For this review, take the finished solid that the model builds, in its own axes (mm). Face numbers are marked on the shaded views. Round coordinates to 2 decimals unless told otherwise and drop trailing zeros. Loops run counter-clockwise (first coordinate to the right, second up) from the corner with the lowest first, then second, coordinate; pieces in that order, holes last.
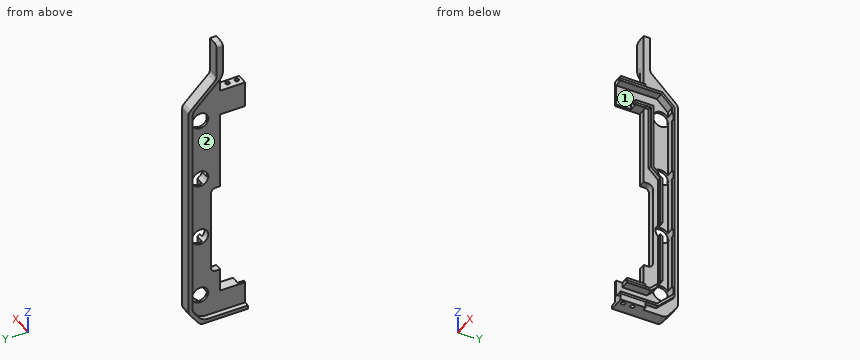
```python
from build123d import *

# Parameters (mm, degrees)
BOSS_EXTRUDE1_DEPTH          = 25
CUT_EXTRUDE1_DEPTH           = 4
FILLET1_R                    = 4
FILLET2_R                    = 10
FILLET3_R                    = 5
FILLET4_R                    = 3
BOSS_EXTRUDE2_DEPTH          = 3
BOSS_EXTRUDE2_DEPTH_BACK     = 3
FILLET5_R                    = 3
SKETCH6_W                    = 13
SKETCH6_H                    = 14
BOSS_EXTRUDE3_DEPTH          = 20
BOSS_EXTRUDE4_DEPTH          = 20
SKETCH9_W                    = 13
SKETCH9_H                    = 2
BOSS_EXTRUDE5_DEPTH          = 8
SKETCH7_W                    = 13
SKETCH7_H                    = 2
CUT_EXTRUDE2_DEPTH           = 5
SKETCH11_R                   = 1.6
CUT_EXTRUDE3_DEPTH           = 19
CUT_EXTRUDE4_START           = -2
SKETCH12_R                   = 1.6
CUT_EXTRUDE4_DEPTH           = 2
CUT_EXTRUDE5_DEPTH           = 6.5
CUT_EXTRUDE5_DEPTH_BACK      = 6.5
CUT_EXTRUDE7_DEPTH           = 247.814201374
BOSS_EXTRUDE6_DEPTH          = 6.5
BOSS_EXTRUDE8_DEPTH          = 3.5
MAKE_THIS_A_SQUARE_OR_SMTH_R = 6.5
CUT_EXTRUDE8_DEPTH           = 134.148413434


with BuildPart() as part:
    # Sketch1 → Boss-Extrude1 (new body)
    with BuildSketch(Plane(origin=(0, 0, 0), x_dir=(0, 0, -1), z_dir=(1, 0, 0))):
        Polygon((0, 0), (-130, 0), (-130, 5), (-100.000366453, 5.148280317), (-77.868517379, 27.5), (101.088229162, 27.5), (114, 18), (114, 0), (74, 0), (74, 7.5), (0, 7.5), align=None)
    extrude(amount=BOSS_EXTRUDE1_DEPTH)

    # Sketch4 → Cut-Extrude1 (cut)
    with BuildSketch(Plane(origin=(25, 0, 0), x_dir=(0, 0, -1), z_dir=(1, 0, 0))):
        Polygon((-100.876178749, 0), (0, 0), (111, 0), (111, 3), (111, 16.482758557), (100.103496394, 24.5), (-76.617181678, 24.5), align=None)
    cut_extrude1 = extrude(amount=-CUT_EXTRUDE1_DEPTH, mode=Mode.SUBTRACT)

    # Mirror2: Cut-Extrude1 across plane
    add(cut_extrude1.mirror(Plane(origin=(12.5, 0, 0), x_dir=(0, 0, 1), z_dir=(1, 0, 0))), mode=Mode.SUBTRACT)

    # Fillet1
    fillet1_edges = [part.edges().sort_by_distance(p)[0] for p in [
        (12.5, 7.5, -74),
        (12.5, 7.5, 0),
    ]]
    fillet(fillet1_edges, radius=FILLET1_R)

    # Fillet2
    fillet2_edges = [part.edges().sort_by_distance(p)[0] for p in [
        (23, 0, 100.876178749),
        (23, 24.5, 76.617181678),
        (23, 24.5, -100.103496394),
        (23, 16.482758557, -111),
        (2, 0, 100.876178749),
        (2, 16.482758557, -111),
        (2, 24.5, -100.103496394),
        (2, 24.5, 76.617181678),
    ]]
    fillet(fillet2_edges, radius=FILLET2_R)

    # Fillet3
    fillet3_edges = [part.edges().sort_by_distance(p)[0] for p in [
        (12.5, 5.148280317, 100.000366453),
        (12.5, 27.5, 77.868517379),
        (12.5, 27.5, -101.088229162),
        (12.5, 18, -114),
    ]]
    fillet(fillet3_edges, radius=FILLET3_R)

    # Fillet4
    fillet4_edges = [part.edges().sort_by_distance(p)[0] for p in [
        (0, 2.5, 130),
        (25, 2.5, 130),
    ]]
    fillet(fillet4_edges, radius=FILLET4_R)

    # Sketch5 → Boss-Extrude2 (add, two sides: drawn at the far end of the back side and taken through both)
    with BuildSketch(Plane(origin=(12.5, 0, 0), x_dir=(0, 0, -1), z_dir=(1, 0, 0)).offset(-BOSS_EXTRUDE2_DEPTH_BACK)):
        Polygon((-117.8659777, 5.059975288), (-103.793914836, 19.271838176), (-72.605250228, 19.271838176), (-95.8659777, 5.059975288), align=None)
    extrude(amount=BOSS_EXTRUDE2_DEPTH + BOSS_EXTRUDE2_DEPTH_BACK)

    # Fillet5
    fillet5_edges = [part.edges().sort_by_distance(p)[0] for p in [
        (12.5, 19.271838176, 103.793914836),
    ]]
    fillet(fillet5_edges, radius=FILLET5_R)

    # Sketch6 → Boss-Extrude3 (add)
    with BuildSketch(Plane.XZ):
        Polygon((0, -111), (4, -111), (4, -93), (21, -93), (21, -111), (25, -111), (25, -114), (0, -114), align=None)
        with Locations((12.5, -102)):
            Rectangle(SKETCH6_W, SKETCH6_H, mode=Mode.SUBTRACT)
    extrude(amount=BOSS_EXTRUDE3_DEPTH)

    # Sketch8 → Boss-Extrude4 (add)
    with BuildSketch(Plane.XZ):
        Polygon((21, 85), (4, 85), (4, 64), (6, 64), (6, 83), (19, 83), (19, 64), (21, 64), align=None)
    extrude(amount=BOSS_EXTRUDE4_DEPTH)

    # Sketch9 → Boss-Extrude5 (add)
    with BuildSketch(Plane.XZ):
        with Locations((12.5, 65)):
            Rectangle(SKETCH9_W, SKETCH9_H)
    extrude(amount=BOSS_EXTRUDE5_DEPTH)

    # Sketch7 → Cut-Extrude2 (cut)
    with BuildSketch(Plane.XZ.offset(20)):
        with Locations((12.5, -94)):
            Rectangle(SKETCH7_W, SKETCH7_H)
    extrude(amount=-CUT_EXTRUDE2_DEPTH, mode=Mode.SUBTRACT)

    # Sketch11 → Cut-Extrude3 (cut)
    with BuildSketch(Plane(origin=(0, 0, -114), x_dir=(-1, 0, 0), z_dir=(0, 0, -1))):
        with Locations((-15.75, -16.25)):
            Circle(SKETCH11_R)
        with Locations((-15.75, -8.75)):
            Circle(SKETCH11_R)
        with Locations((-9.25, -8.75)):
            Circle(SKETCH11_R)
        with Locations((-9.25, -16.25)):
            Circle(SKETCH11_R)
    extrude(amount=-CUT_EXTRUDE3_DEPTH, mode=Mode.SUBTRACT)

    # Sketch12 → Cut-Extrude4 (cut)
    with BuildSketch(Plane.XY.offset(85).offset(CUT_EXTRUDE4_START)):
        with Locations(Location((15.75, -16.25, 0), (0, 0, 180))):
            Circle(SKETCH12_R)
        with Locations(Location((9.25, -16.25, 0), (0, 0, 180))):
            Circle(SKETCH12_R)
        with Locations(Location((9.25, -8.75, 0), (0, 0, 180))):
            Circle(SKETCH12_R)
        with Locations(Location((15.75, -8.75, 0), (0, 0, 180))):
            Circle(SKETCH12_R)
    extrude(amount=CUT_EXTRUDE4_DEPTH, mode=Mode.SUBTRACT)

    # Sketch14 → Cut-Extrude5 (cut, two sides: drawn at the far end of the back side and taken through both)
    with BuildSketch(Plane(origin=(12.5, 0, 0), x_dir=(0, 0, -1), z_dir=(1, 0, 0)).offset(-CUT_EXTRUDE5_DEPTH_BACK)):
        Polygon((-83, 0), (-83, 13.475167258), (-72.975167258, 23.5), (95.592427597, 23.5), (109, 10.092427597), (109, 0), (95, 0), (95, 3.57939317), (87.07939317, 11.5), (-5.825100808, 11.5), (-13.325100808, 4), (-66, 4), (-66, 0), align=None)
    extrude(amount=CUT_EXTRUDE5_DEPTH + CUT_EXTRUDE5_DEPTH_BACK, mode=Mode.SUBTRACT)

    # Sketch17 → Cut-Extrude7 (cut, through all)
    with BuildSketch(Plane.XY.offset(130)):
        Polygon((12.5, -20), (25, -20), (25, 27.5), (9.5, 27.5), (9.5, 5.138043697), (9.5, 0), (12.5, 0), align=None)
    extrude(amount=-CUT_EXTRUDE7_DEPTH, mode=Mode.SUBTRACT)

    # Sketch18 → Boss-Extrude6 (add)
    with BuildSketch(Plane(origin=(6, 0, 0), x_dir=(0, 0, -1), z_dir=(1, 0, 0))):
        Polygon((-66.15, -8), (-68.15, -8), (-68.15, 6.15), (-14.215659968, 6.15), (-6.715659968, 13.65), (87.96995233, 13.65), (97.15, 4.46995233), (97.15, -15), (95.15, -15), (95.15, 3.641525205), (87.141525205, 11.65), (-5.887232843, 11.65), (-13.387232843, 4.15), (-66.15, 4.15), align=None)
        Polygon((-82.85, -20), (-82.85, 13.413035223), (-72.913035223, 23.35), (95.530295563, 23.35), (108.85, 10.030295563), (108.85, -20), (106.85, -20), (106.85, 9.201868438), (94.701868438, 21.35), (-72.084608099, 21.35), (-80.85, 12.584608099), (-80.85, -20), align=None)
    extrude(amount=BOSS_EXTRUDE6_DEPTH)

    # Sketch24 → Boss-Extrude8 (add)
    with BuildSketch(Plane(origin=(6, 0, 0), x_dir=(0, 0, -1), z_dir=(1, 0, 0))):
        Polygon((-83, -20), (-82.85, -20), (-82.85, 13.413035223), (-72.913035223, 23.35), (95.530295563, 23.35), (108.85, 10.030295563), (108.85, -20), (109, -20), (109, 10.092427597), (95.592427597, 23.5), (-72.975167258, 23.5), (-83, 13.475167258), align=None)
        Polygon((-66.15, -8), (-66, -8), (-66, 4), (-13.325100808, 4), (-5.825100808, 11.5), (87.07939317, 11.5), (95, 3.57939317), (95, -15), (95.15, -15), (95.15, 3.641525205), (87.141525205, 11.65), (-5.887232843, 11.65), (-13.387232843, 4.15), (-66.15, 4.15), align=None)
    extrude(amount=BOSS_EXTRUDE8_DEPTH)

    # MAKE THIS A SQUARE OR SMTH → Cut-Extrude8 (cut, through all)
    with BuildSketch(Plane.ZY.offset(-4)):
        with Locations((-91, 16)):
            Circle(MAKE_THIS_A_SQUARE_OR_SMTH_R)
        with Locations((-39.333333333, 16)):
            Circle(MAKE_THIS_A_SQUARE_OR_SMTH_R)
        with Locations(Location((64, 16, 0), (0, 0, 55.394002372))):
            Circle(MAKE_THIS_A_SQUARE_OR_SMTH_R)
        with Locations(Location((12.333333333, 16, 0), (0, 0, 55.394002372))):
            Circle(MAKE_THIS_A_SQUARE_OR_SMTH_R)
    extrude(amount=-CUT_EXTRUDE8_DEPTH, mode=Mode.SUBTRACT)


solid = part.part
```
(1) Insertion check: pin 1 Ø12 at (y, z) = (22.5, -61) entering from -X; pin 2 Ø2 at (x, z) = (11, 64.5) entering from +Y; pin 3 Ø1.6 at (x, z) = (7, -84.5) entering from -Y; pin 4 Ø3 at (y, z) = (-10.5, 62) entering from -X. Each pin has a flat end and moves straight along its axis. Give the tip position at first contact, or say it passes through.
(2) The part is to be moulded in two halves that separate along Z. For the marked faces 1 and 2, say which applies: pulls with the +Z half, pulls with the -Z half, needs draft (parallel to the pull), parting line crosses it, or undercut.
(3) Add section A-A (z = -49). Give the boundary of the cut face in (x, y), plus the area to 3 significant figures.
(4) For L1, parallel to X at y = -16, z = 84; L2, parallel to Y at x = 9.25, z = 21; L3, parallel to Z at x = 5.5, y = -3, list the stretches that pass through material, from the lowest coordinate up.
Outcome:
1. pin 1: stops at x = 0
1. pin 2: stops at y = 23.35
1. pin 3: stops at y = 0
1. pin 4: passes through
2. face 1: undercut
2. face 2: undercut
3. outline: (0, 24.5) - (4, 24.5) - (4, 7.5) - (9.5, 7.5) - (9.5, 11.65) - (12.5, 11.65) - (12.5, 13.65) - (6, 13.65) - (6, 21.35) - (12.5, 21.35) - (12.5, 23.35) - (9.5, 23.35) - (9.5, 27.5) - (0, 27.5) - close
3. area: 107 mm2
4. L1: x = 4 to 7.67, 10.83 to 12.5
4. L2: y = 0 to 6.15, 21.35 to 27.5
4. L3: z = -114 to -93, 64 to 85
